Here's how the part is built. I have some questions about the finished solid (model axes, mm). A direction names the side the tool comes from. Give positions to 0.01 mm unless a question says otherwise; leave off trailing zeros. Loops run counter-clockwise (first coordinate to the right, second up) from the corner with the lowest first, then second, coordinate; pieces in that order, holes last.
Q1. If we section it at B-B (x = 3.5): Please give me the cut outline in (y, z), plus the area to 3 significant figures.
Q2. Will these pins go through, and if not, where does the flat tip stop? P1, Ø2, axis at x = 16, z = -4, coming from the +Y side; P2, Ø1.7, axis at y = 2, z = 0.5, coming from the -X side; P3, Ø2, axis at x = 14, y = -0.5, coming from the +Z side.
Q3. I need wall thicknesses on line 1 (X direction, y = 2, z = 4); line 2 (Y direction, x = 21.5, z = 2); line 3 (Z direction, x = -0.5, y = -0.25). Which ranges of each line are inside material? Lowest first, please.
Q4. We'd pull the mould along Z, two halves only. Please class faces 6 (the face through (0, 3, -3)), 7 (the face through (-3.55, -5.158, -3.955)), 8 (the face through (-2.57, -0.11, 0.51)): +Z half, -Z half, draft (parallel to the pull), parting line (faces both ways), or undercut.
Q5. For faces 1 (the face through (-4, 3.15, 0.24)), 2 (the face through (24, 0, 0)), 3 (the face through (15.92, -0.867, -3.905)), 4 (the face through (-8, 2.5, -2.5)), 5 (the face through (3.922, 3.34, -1.385)), which set-ups out of +Z, -Z, +X, -X, +Y, -Y let a thin tool reach every point of the face, with its end or its side?
Q6. If we section it at A-A (x = -3): Please give me the cut outline in (y, z).
Q7. If we section it at C-C (x = 10): Please give me the cut outline in (y, z), plus the area to 3 significant figures.
Autodesk Inventor part; units mm, degrees
ref_plane "bolt_to_plane_washer_XY" through (5.6, 0, 0) normal (1, 0, 0) x (0, 0, -1)
ref_plane "bolt_to_plane_washer_YZ" through (5.6, 0, 0) normal (0, 0, -1) x (0, 1, 0)
ref_plane "bolt_to_plane_washer_ZX" through (5.6, 0, 0) normal (0, 1, 0) x (1, 0, 0)
sketch "Sketch_6" plane through (0, 0, 0) normal (0, 0, 1) x (1, 0, 0)
  line L0 (24, 0) -> (7.0715, 0)
  line L1 (7.0715, 0) -> (7.0715, 3.233)
  line L2 (7.0715, 3.233) -> (8.4, 4)
  line L3 (8.4, 4) -> (23.233, 4)
  line L4 (23.233, 4) -> (24, 3.233)
  line L5 (24, 3.233) -> (24, 0)
  line L6 (24, 0) -> (7.0715, 0)
revolve "Revolution1" add sketch "Sketch_6" angle 360 about axis through (24, 0, 0) along (1, 0, 0)
thread "Thread1"
sketch "Sketch_1" plane through (0, 0, 0) normal (0, 0, 1) x (1, 0, 0)
  line L0 (8.4, 0) -> (-8, 0)
  line L1 (-2.2679, 0) -> (-4, 3)
  line L2 (-4, 3) -> (-8, 3)
  line L3 (-8, 3) -> (-8, 5.7)
  line L4 (-8, 5.7) -> (-7.2, 6.5)
  line L5 (-7.2, 6.5) -> (0, 6.5)
  line L6 (0, 6.5) -> (0, 3.616)
  line L7 (0, 3.616) -> (8.4, 3.616)
  line L8 (8.4, 3.616) -> (8.4, 0)
  line L9 (8.4, 0) -> (-2.2679, 0)
revolve "Revolution2" add sketch "Sketch_1" angle 360 about axis through (8.4, 0, 0) along (1, 0, 0)
sketch "Sketch_2" plane through (-8, 0, 0) normal (1, 0, 0) x (0, 0, -1)
  line L0 (-3, -1.7321) -> (0, -3.4641)
  line L1 (0, -3.4641) -> (3, -1.7321)
  line L2 (3, -1.7321) -> (3, 1.7321)
  line L3 (3, 1.7321) -> (0, 3.4641)
  line L4 (0, 3.4641) -> (-3, 1.7321)
  line L5 (-3, 1.7321) -> (-3, -1.7321)
extrude "Extrusion1" cut sketch "Sketch_2" along normal blind 4
ref_plane "bolt_to_plane_washer_XY" through (5.6, 0, 0) normal (1, 0, 0) x (0, 0, -1)
ref_plane "bolt_to_plane_washer_YZ" through (5.6, 0, 0) normal (0, 0, -1) x (0, 1, 0)
ref_plane "bolt_to_plane_washer_ZX" through (5.6, 0, 0) normal (0, 1, 0) x (1, 0, 0)
ref_plane "bolt_to_spring_washer_XY" through (2.8, 0, 0) normal (1, 0, 0) x (0, 0, -1)
ref_plane "bolt_to_spring_washer_YZ" through (2.8, 0, 0) normal (0, 0, -1) x (0, 1, 0)
ref_plane "bolt_to_spring_washer_ZX" through (2.8, 0, 0) normal (0, 1, 0) x (1, 0, 0)
ref_plane "screw_to_body_XY" through (0, 0, 0) normal (1, 0, 0) x (0, 0, -1)
ref_plane "screw_to_body_YZ" through (0, 0, 0) normal (0, 0, -1) x (0, 1, 0)
ref_plane "screw_to_body_ZX" through (0, 0, 0) normal (0, 1, 0) x (1, 0, 0)
ref_plane "to_washer_XY" through (24, 0, 0) normal (1, 0, 0) x (0, 0, -1)
ref_plane "to_washer_YZ" through (24, 0, 0) normal (0, 0, -1) x (0, 1, 0)
ref_plane "to_washer_ZX" through (24, 0, 0) normal (0, 1, 0) x (1, 0, 0)
properties part number "HCBST8-24_Screw"
Check sheet entries:
1. outline: circle Ø7.23 at (0, 0)
1. area: 41.1 mm2
2. P1: stops at y = 2.65
2. P2: stops at x = -3.95
2. P3: stops at z = 4
3. line 1: x = -8 to 0
3. line 2: y = -3.46 to 3.46
3. line 3: z = -6.5 to 6.5
4. face 6: draft
4. face 7: parting line
4. face 8: undercut
5. face 1: -X
5. face 2: +Z, -Z, +X, +Y, -Y
5. face 3: +X
5. face 4: +Z, -Z, -X, +Y, -Y
5. face 5: none
6. outline: circle Ø13 at (0, 0); hole circle Ø2.54 at (0, 0)
7. outline: circle Ø8 at (0, 0)
7. area: 50.3 mm2
